Design review of the part built by this model. Coordinates are the model's own, in mm. A direction names the side the tool comes from. Coordinates: 2 decimals unless noted, no trailing zeros. Loops run counter-clockwise (first coordinate to the right, second up) from the corner with the lowest first, then second, coordinate; pieces in that order, holes last. Notation, with made-up numbers: (27.25, 24) -> (50.25, 24) arc R17 ccw to (50.25, 38) -> close; hole circle Ø10 at (33.25, -15.5). An arc over 180 degrees is marked (long way). Answer as a JSON object with one key per item and string values.
Autodesk Inventor part; units mm, degrees
ref_plane "YZ Plane" through (0, 0, 0) normal (1, 0, 0) x (0, 1, 0)
ref_plane "XZ Plane" through (0, 0, 0) normal (0, 1, 0) x (-1, 0, 0)
ref_plane "XY Plane" through (0, 0, 0) normal (0, 0, 1) x (1, 0, 0)
sketch "Sketch1" plane through (0, 0, 0) normal (0, 1, 0) x (-1, 0, 0)
  circle A0 centre (0, 0) radius 23.725
  circle A1 centre (0, 0) radius 13.725
  dimension "d0" = 47.45
  dimension "d1" = 27.45
extrude "Extrusion1" add sketch "Sketch1" along normal blind 2
sketch "Sketch2" plane through (0, 2, 0) normal (0, 1, 0) x (1, 0, 0)
  line L0 (-28.725, -1) -> (-18.725, -1)
  line L1 (-18.725, -1) -> (-18.725, 1)
  line L2 (-18.725, 1) -> (-28.725, 1)
  line L3 (-28.725, 1) -> (-28.725, -1)
  point P0 (0, 0)
  dimension "d4" = 1
  dimension "d5" = 2
  dimension "d6" = 18.725
  dimension "d7" = 10
extrude "Extrusion2" cut sketch "Sketch2" against normal blind 2
pattern_circular "Circular Pattern1" count 6 over 360 about axis through (0, -10, 0) along (0, 1, 0) of "Extrusion2"
sketch "Sketch3" plane through (0, 2, 0) normal (0, 1, 0) x (1, 0, 0)
  circle A0 centre (-8.6603, -5) radius 6
  line L0 (-8.6603, -5) -> (0, 0) construction
  line L1 (-33.1855, 0) -> (33.1855, 0)
  dimension "d13" = 30
  dimension "d14" = 5
  dimension "d15" = 12
extrude "Extrusion3" cut sketch "Sketch3" against normal blind 2
pattern_circular "Circular Pattern2" count 6 over 360 about axis through (0, -10, 0) along (0, 1, 0) of "Extrusion3"
properties part number "Ring_n3"
1) Add section A-A, the plane z = -19. Give the boundary of the cut face in (x, y).
Completed:
{"outline": "(-14.21, 0) -> (-12.12, 0) -> (-12.12, 2) -> (-14.21, 2) -> close; (-9.81, 0) -> (9.81, 0) -> (9.81, 2) -> (-9.81, 2) -> close; (12.12, 0) -> (14.21, 0) -> (14.21, 2) -> (12.12, 2) -> close"}
2) Wall thickness on probe 1 along X at (y, z) = (1.45, 18); probe 2 along Z at (x, y) = (14, 1.6); probe 3 along X at (y, z) = (1.7, 19.5): over which ranges is each line inside the solid? List them lowest first.
Completed:
{"probe 1": "-15.46 to -11.55, -9.24 to 9.24, 11.55 to 15.46", "probe 2": "-19.15 to -7.74, -2.26 to 2.26, 7.74 to 19.15", "probe 3": "-13.51 to -12.41, -10.1 to 10.1, 12.41 to 13.51"}
3) The part is to be moulded in two halves that separate along Z. For faces 1 (the cylindrical face through (-0.16, 0.986, -23.724)), 2 (the cylindrical face through (-20.466, 0.986, 12.001)), 3 (the cylindrical face through (6.84, 0.99, -11.9)), say which applies: pulls with the +Z half, pulls with the -Z half, needs draft (parallel to the pull), parting line crosses it, or undercut.
Completed:
{"face 1": "pulls with the -Z half", "face 2": "pulls with the +Z half", "face 3": "undercut"}
4) Add section B-B, the plane x = 12. Give the boundary of the cut face in (y, z), and give its area (3 significant figures).
Completed:
{"outline": "(0, -18.78) -> (2, -18.78) -> (2, -9.98) -> (0, -9.98) -> close; (0, 9.98) -> (2, 9.98) -> (2, 18.78) -> (0, 18.78) -> close", "area": "35.2 mm²"}
5) Add section C-C, the plane z = 4.5. Give the boundary of the cut face in (x, y), and give its area (3 significant figures).
Completed:
{"outline": "(-23.29, 0) -> (-14.64, 0) -> (-14.64, 2) -> (-23.29, 2) -> close; (14.64, 0) -> (23.29, 0) -> (23.29, 2) -> (14.64, 2) -> close", "area": "34.6 mm²"}
6) For faces 4 (the flat face through (9.35, 1.014, -16.223)), 5 (the flat face through (21, 1, 1)), 6 (the cylindrical face through (20.466, 0.986, -12.001)), list the 3-axis set-ups (+Z, -Z, +X, -X, +Y, -Y) from which the entire face can be reached by the end or side of a thin tool; tool diameter is ignored.
Completed:
{"face 4": "+Y, -Y", "face 5": "+X, +Y, -Y", "face 6": "-Z, +X, +Y, -Y"}
7) Clearance check with flat-ended pins moving along their axes: pin 1 Ø1 at (y, z) = (1.5, 0) entering from +X (3 decimals); pin 2 Ø1 at (x, y) = (-20.5, 0.5) entering from -Z; pin 3 Ø0.6 at (y, z) = (1, -0.5) entering from -X (3 decimals). State where each tip first meets the part, or that it passes through.
Completed:
{"pin 1": "x = 18.725", "pin 2": "z = -12.76", "pin 3": "x = -18.725"}
8) Add section D-D, the plane x = -15.5. Give the boundary of the cut face in (y, z).
Completed:
{"outline": "(0, -17.96) -> (2, -17.96) -> (2, 17.96) -> (0, 17.96) -> close"}
